from build123d import *

# Parameters (mm, degrees)
F0_R           = 12.5
F1_DEPTH       = 30
F2_R           = 3
F4_D           = 6
F4_CBORE_D     = 10
F4_CBORE_DEPTH = 10


with BuildPart() as f1:
    # F0 (on Right) → F1 (new body)
    with BuildSketch(Plane.YZ):
        Circle(F0_R)
    extrude(amount=F1_DEPTH)

    # F2
    f2_edges = [f1.edges().sort_by_distance(p)[0] for p in [
        (30, -12.5, 0),
    ]]
    fillet(f2_edges, radius=F2_R)

    # F4 (through all)
    with Locations(Plane.YZ.offset(30)):
        with Locations((0, 0)):
            CounterBoreHole(F4_D / 2, F4_CBORE_D / 2, F4_CBORE_DEPTH)


solid = f1.part
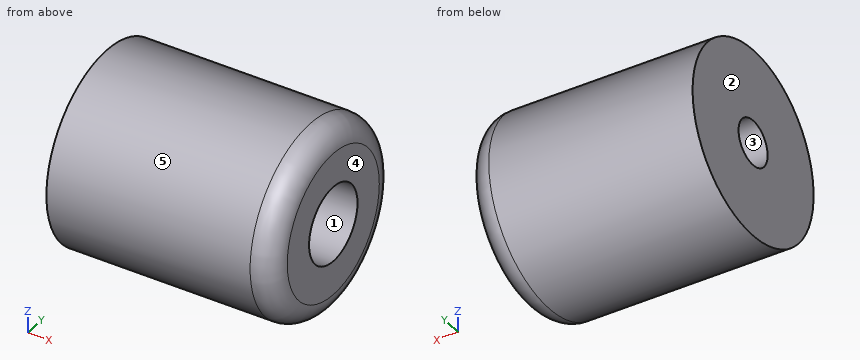
The listing builds one solid part. Answer for the finished solid, in the listing's coordinates (mm). Face numbers are marked on the shaded views. A direction names the side the tool comes from. Give positions to 0.01 mm unless a question says otherwise; leave off trailing zeros. Write each loop counter-clockwise with the first axis right and the second up, starting at its lowest first coordinate (ties: lowest second). Pieces come first, ordered by that corner, then holes.
Item 1: Flat-ended cylindrical pins translate along their axes: P1, Ø5, axis at x = 7.5, z = 4, coming from the +Y side; P2, Ø5.5, axis at y = 0, z = 0, coming from the +X side; P3, Ø6, axis at x = 6, z = -6.5, coming from the -Y side; P4, Ø2, axis at x = 22, y = -7.5, coming from the -Z side. Find the tip coordinate at first contact, or state that the pin passes through.
Item 2: Determine the mould class of the marked faces 3, 4 and 5 for opening direction Y: released by +Y, released by -Y, zero draft, split by the parting line, or undercut.
Item 3: Which of the six approach directions +Z, -Z, +X, -X, +Y, -Y give full straight-line access (tool end or side, diameter ignored) to the marked faces 1 and 2?
Item 4: Find the intervals of material crossed by line 1 along Z through (x, y) = (23.25, 0); line 2 along Y through (x, z) = (20.5, -0.25); line 3 along Z through (x, y) = (10, 0), in increasing order.
Item 5: Section C-C, the plane x = 18.5 is taken. Write down the section's boundary in (y, z), plus the area to 3 significant figures.
Item 6: Section A-A, the plane y = 0 is taken. Write down the section's boundary in (x, z), plus the area to 3 significant figures.
Completed:
1. P1: stops at y = 12.41
1. P2: passes through
1. P3: stops at y = -12
1. P4: stops at z = -10.68
2. face 3: undercut
2. face 4: zero draft
2. face 5: split by the parting line
3. face 1: +X
3. face 2: +Z, -Z, -X, +Y, -Y
4. line 1: z = -12.5 to -5, 5 to 12.5
4. line 2: y = -12.5 to -4.99, 4.99 to 12.5
4. line 3: z = -12.5 to -3, 3 to 12.5
5. outline: circle Ø25 at (0, 0); hole circle Ø6 at (0, 0)
5. area: 463 mm2
6. outline: (0, -12.5) - (27, -12.5) arc R3 ccw to (30, -9.5) - (30, -5) - (20, -5) - (20, -3) - (0, -3) - close; (0, 3) - (20, 3) - (20, 5) - (30, 5) - (30, 9.5) arc R3 ccw to (27, 12.5) - (0, 12.5) - close
6. area: 526 mm2
